from build123d import *

# Parameters (mm, degrees)
F0_W     = 24
F0_H     = 126
F0_W_2   = 16
F0_H_2   = 112
F1_DEPTH = 24.5
F2_DEPTH = 2
F3_R     = 1.85
F4_DEPTH = 6
F5_R     = 6
F6_R     = 2
F7_DEPTH = 1.5
F8_R     = 1


with BuildPart() as f1:
    # F0 (on Front) → F1 (new body)
    with BuildSketch(Plane.XZ):
        Rectangle(F0_W, F0_H)
        Rectangle(F0_W_2, F0_H_2, mode=Mode.SUBTRACT)
    extrude(amount=F1_DEPTH)

    # F0 (on Front) → F2 (join)
    with BuildSketch(Plane.XZ):
        Rectangle(F0_W_2, F0_H_2)
    extrude(amount=F2_DEPTH)

    # F3 (on face) → F4 (join)
    with BuildSketch(Plane.XZ.offset(24.5)):
        with BuildLine():
            ThreePointArc((0, 57.65), (1.3081475452, 58.1918524548), (1.85, 59.5))
            ThreePointArc((1.85, 59.5), (1.3081475452, 60.8081475452), (0, 61.35))
            Line((0, 61.35), (0, 57.65))
        make_face()
        with BuildLine():
            Line((0, 57.65), (0, 61.35))
            ThreePointArc((0, 61.35), (-1.85, 59.5), (0, 57.65))
        make_face()
        with Locations((0, -59.5)):
            Circle(F3_R)
    extrude(amount=F4_DEPTH)

    # F5
    f5_edges = [f1.edges().sort_by_distance(p)[0] for p in [
        (-12, -12.25, -63),
        (-12, -12.25, 63),
    ]]
    fillet(f5_edges, radius=F5_R)

    # F6 (on Front) → F7 (join)
    with BuildSketch(Plane.XZ):
        with BuildLine():
            Line((6.5, 63), (6.5, 68.3245120645))
            ThreePointArc((6.5, 68.3245120645), (0, 74.8245120645), (-6.5, 68.3245120645))
            Line((-6.5, 68.3245120645), (-6.5, 63))
            Line((-6.5, 63), (-6, 63))
            Line((-6, 63), (6.5, 63))
        make_face()
        with Locations((0, 68.3245120645)):
            Circle(F6_R, mode=Mode.SUBTRACT)
        with BuildLine():
            ThreePointArc((-6.5, 62.9791303716), (-6.2502176759, 62.9947803225), (-6, 63))
            Line((-6, 63), (-6.5, 63))
            Line((-6.5, 63), (-6.5, 62.9791303716))
        make_face()
        with BuildLine():
            ThreePointArc((-6.5, -68.3245120645), (0, -74.8245120645), (6.5, -68.3245120645))
            Line((6.5, -68.3245120645), (6.5, -63))
            Line((6.5, -63), (-6, -63))
            ThreePointArc((-6, -63), (-6.2502176759, -62.9947803225), (-6.5, -62.9791303716))
            Line((-6.5, -62.9791303716), (-6.5, -68.3245120645))
        make_face()
        with Locations((0, -68.3245120645)):
            Circle(F6_R, mode=Mode.SUBTRACT)
    extrude(amount=F7_DEPTH)

    # F8
    f8_edges = [f1.edges().sort_by_distance(p)[0] for p in [
        (-1.85, -30.5, 59.5),
        (-1.85, -30.5, -59.5),
    ]]
    fillet(f8_edges, radius=F8_R)


solid = f1.part
Work out the finished part from the listing and answer in its coordinate system (mm). A direction names the side the tool comes from. Give positions to 0.01 mm unless a question says otherwise; leave off trailing zeros. Loops run counter-clockwise (first coordinate to the right, second up) from the corner with the lowest first, then second, coordinate; pieces in that order, holes last. Notation, with made-up numbers: (-36, 1.5) -> (13, 1.5) arc R29 ccw to (13, 34.5) -> close; hole circle Ø3 at (11.25, 63). An arc over 180 degrees is marked (long way). Use a Markdown table: item, result. Add a question column.
1) Consider line 1 along Z through (x, y) = (0, -0.65); line 2 along X through (y, z) = (-24, -9.5); line 3 along Z through (x, y) = (-6.75, -17). Determine where each line is inside the solid, lowest interval first.
2) Which of the six approach directions +Z, -Z, +X, -X, +Y, -Y give full straight-line access (tool end or side, diameter ignored) to faces 1 (the flat face through (0, 0, 1)), 2 (the flat face through (0, -13, -56)), 3 (the flat face through (-2, -1.5, 70))?
3) Each of these flat-tipped pins is pushed along its axis until it touches: P1, Ø8, axis at x = 0, y = -15, coming from the -Z side; P2, Ø1.6, axis at y = -0.5, z = -64.5, coming from the -X side; P3, Ø1.5, axis at x = 9, z = 57.5, coming from the -Y side. Where does it stop, or does it pass through?
4) The part is cut by section B-B, the plane z = 2. Determine the outline of the cut face in (x, y).
5) For a pull along Z with two mould halves and no side action, classify faces 4 (the flat face through (8, -13, -1)), 5 (the flat face through (-8, -13, -1)), 6 (the flat face through (0, -1.5, -66)), 7 (the cylindrical face through (0.143, -0.74, 74.823)) as +Z half, -Z half, draft (parallel to the pull), parting line (faces both ways), or undercut.
6) The part is cut by section C-C, the plane y = -26. Determine the outline of the cut face in (x, z), plus the area to 3 significant figures.
7) The part is cut by section D-D, the plane x = 3.5. Determine the outline of the cut face in (y, z).
8) The part is cut by section A-A, the plane y = -20.5. Determine the outline of the cut face in (x, z), plus the area to 3 significant figures.
Reported:
| question | item | result |
|---|---|---|
| 1 | line 1 | z = -74.82 to -70.32, -66.32 to 66.32, 70.32 to 74.82 |
| 1 | line 2 | x = -12 to -8, 8 to 12 |
| 1 | line 3 | z = -62.95 to -56, 56 to 62.95 |
| 2 | face 1 | +Z, -Z, +X, -X, +Y |
| 2 | face 2 | -Y |
| 2 | face 3 | +Z, +X, -X, -Y |
| 3 | P1 | stops at z = -63 |
| 3 | P2 | stops at x = -6.5 |
| 3 | P3 | stops at y = -24.5 |
| 4 | outline | (-12, -24.5) -> (-8, -24.5) -> (-8, -2) -> (8, -2) -> (8, -24.5) -> (12, -24.5) -> (12, 0) -> (-12, 0) -> close |
| 5 | face 4 | undercut |
| 5 | face 5 | undercut |
| 5 | face 6 | draft |
| 5 | face 7 | +Z half |
| 6 | outline | circle Ø3.7 at (0, -59.5); circle Ø3.7 at (0, 59.5) |
| 6 | area | 21.5 mm^2 |
| 7 | outline | (-24.5, -63) -> (-1.5, -63) -> (-1.5, -73.8) -> (0, -73.8) -> (0, 73.8) -> (-1.5, 73.8) -> (-1.5, 63) -> (-24.5, 63) -> (-24.5, 56) -> (-2, 56) -> (-2, -56) -> (-24.5, -56) -> close |
| 8 | outline | (-12, -57) arc R6 ccw to (-6, -63) -> (12, -63) -> (12, 63) -> (-6, 63) arc R6 ccw to (-12, 57) -> close; hole (-8, -56) -> (8, -56) -> (8, 56) -> (-8, 56) -> close |
| 8 | area | 1,220 mm^2 |
